Verification items for the finished model (mm, model axes). Face numbers are marked on the shaded views. Coordinates: 2 decimals unless noted, no trailing zeros. Order: outer loops, then holes, each group sorted by start corner. A loop starts at its lowest first (then second) coordinate and runs counter-clockwise, first axis right, second up.
Q1. Draft check along Z on the marked faces 1, 2 and 3. Enter one of: pulls with the +Z half, pulls with the -Z half, needs draft (parallel to the pull), parting line crosses it, or undercut.
Q2. Cross-section at C-C, the plane z = 37. Record the boundary of the cut face in (x, y).
Q3. Cross-section at A-A, the plane x = -65. Record the boundary of the cut face in (y, z).
Q4. Cross-section at D-D, the plane z = 49.5. Record the boundary of the cut face in (x, y), and give its area (3 significant figures).
Q5. Depth check by flat-ended pin: P1, Ø3, axis at x = -34.3, z = -2.66, coming from the -Y side; P2, Ø8, axis at x = 31, z = -0.5, coming from the +Y side; P3, Ø12, axis at x = -205.5, y = 4, coming from the +Z side; P4, Ø11.5, axis at x = 32.47, z = -2.66, coming from the -Y side. Enter the tip coordinate at first touch or a pass-through.
Q6. Thickness scan on line 1 (Y direction, x = 15, z = -5.5); line 2 (X direction, y = 1, z = 0); line 3 (Z direction, x = -62.5, y = 11.75). Record the ranges inside material, lowest first.
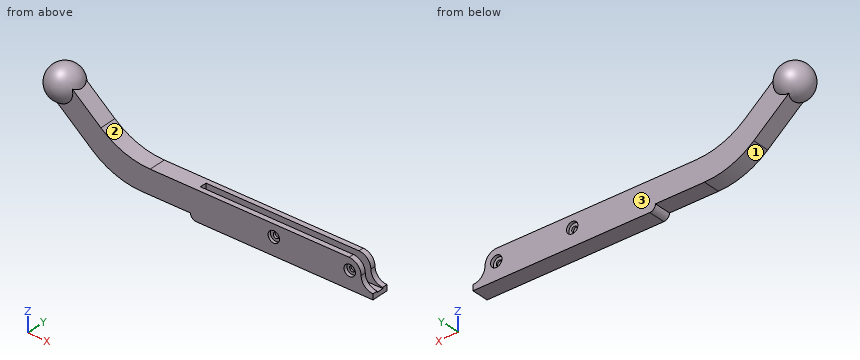
from build123d import *

# Parameters (mm, degrees)
SKETCH_1_W          = 150
SKETCH_1_H          = 21.000000000000004
EXTRUDE_1_DEPTH     = 15
CUT_EXTRUDE_1_DEPTH = 145
SKETCH_3_R          = 5.000000000000004
CUT_EXTRUDE_2_DEPTH = 3
CUT_EXTRUDE_START   = -3
SKETCH_4_R          = 5.000000000000001
CUT_EXTRUDE_3_DEPTH = 3
SKETCH_5_R          = 2.4999999999999987
CUT_EXTRUDE_4_DEPTH = 20
SKETCH_6_R          = 5.000000000000001
CUT_EXTRUDE_5_DEPTH = 20
SKETCH_7_R          = 5.999999999999998
EXTRUDE_2_DEPTH     = 2
SKETCH_8_R          = 6.000000000000003
EXTRUDE_3_DEPTH     = 2
SKETCH_9_R          = 2.500000000000002
CUT_EXTRUDE_6_DEPTH = 20
EXTRUDE_5_DEPTH     = 15
EXTRUDE_6_DEPTH     = 5
FILLET_1_R          = 5
FILLET_2_R          = 10.5
FILLET_3_R          = 67.5
SKETCH_17_W         = 22.000000000000004
SKETCH_17_H         = 5.999999999999995
CUT_EXTRUDE_7_DEPTH = 200


with BuildPart() as part:
    # Sketch 1 → Extrude 1 (new body)
    with BuildSketch(Plane(origin=(0, 0, 0), x_dir=(1, 0, 0), z_dir=(0, 1, 0))):
        with Locations((-32.52921535893155, 2.6552587646076753)):
            Rectangle(SKETCH_1_W, SKETCH_1_H)
    extrude(amount=EXTRUDE_1_DEPTH)

    # Sketch 2 → Cut-Extrude 1 (cut)
    with BuildSketch(Plane(origin=(42.470784641068455, 0, 0), x_dir=(0, 0, -1), z_dir=(1, 0, 0))):
        Polygon((-7.844741235392326, 10.499999999999998), (13.155258764607675, 10.499999999999998), (13.155258764607675, 4.500000000000001), (-7.844741235392326, 4.5), align=None)
    extrude(amount=-CUT_EXTRUDE_1_DEPTH, mode=Mode.SUBTRACT)

    # Sketch 3 → Cut-Extrude 2 (cut)
    with BuildSketch(Plane(origin=(0, 15, 0), x_dir=(1, 0, 0), z_dir=(0, 1, 0))):
        with Locations(Location((32.47078464106845, 2.655258764607675, 0), (0, 0, 270))):
            Circle(SKETCH_3_R)
    extrude(amount=-CUT_EXTRUDE_2_DEPTH, mode=Mode.SUBTRACT)

    # Sketch 4 → Cut-Extrude 3 (cut)
    with BuildSketch(Plane(origin=(0, 0, 0), x_dir=(-1, 0, 0), z_dir=(0, -1, 0)).offset(CUT_EXTRUDE_START)):
        with Locations(Location((-32.47078464106845, 2.655258764607675, 0), (0, 0, 270))):
            Circle(SKETCH_4_R)
    extrude(amount=CUT_EXTRUDE_3_DEPTH, mode=Mode.SUBTRACT)

    # Sketch 5 → Cut-Extrude 4 (cut)
    with BuildSketch(Plane(origin=(0, 3, 0), x_dir=(-1, 0, 0), z_dir=(0, -1, 0))):
        with Locations(Location((-32.47078464106845, 2.655258764607675, 0), (0, 0, 270))):
            Circle(SKETCH_5_R)
    extrude(amount=-CUT_EXTRUDE_4_DEPTH, mode=Mode.SUBTRACT)

    # Sketch 6 → Cut-Extrude 5 (cut)
    with BuildSketch(Plane(origin=(0, 15, 0), x_dir=(1, 0, 0), z_dir=(0, 1, 0))):
        with Locations(Location((-34.295534758931545, 2.655258764607675, 0), (0, 0, 270))):
            Circle(SKETCH_6_R)
    extrude(amount=-CUT_EXTRUDE_5_DEPTH, mode=Mode.SUBTRACT)

    # Sketch 7 → Extrude 2 (add)
    with BuildSketch(Plane(origin=(0, 4.5, 1.9e-16), x_dir=(1, 0, 0), z_dir=(0, 1, 4e-17))):
        with Locations((-34.295534758931545, 2.655258764607675)):
            Circle(SKETCH_7_R)
    extrude(amount=-EXTRUDE_2_DEPTH)

    # Sketch 8 → Extrude 3 (add)
    with BuildSketch(Plane(origin=(0, 10.499999999999998, 0), x_dir=(-1, 0, 0), z_dir=(0, -1, 0))):
        with Locations((34.295534758931545, 2.655258764607675)):
            Circle(SKETCH_8_R)
    extrude(amount=-EXTRUDE_3_DEPTH)

    # Sketch 9 → Cut-Extrude 6 (cut)
    with BuildSketch(Plane(origin=(0, 12.499999999999998, 0), x_dir=(1, 0, 0), z_dir=(0, 1, 0))):
        with Locations(Location((-34.295534758931545, 2.655258764607675, 0), (0, 0, 270))):
            Circle(SKETCH_9_R)
    extrude(amount=-CUT_EXTRUDE_6_DEPTH, mode=Mode.SUBTRACT)



with BuildPart() as body_2:
    # Sketch 12 → Extrude 5 (new body)
    with BuildSketch(Plane(origin=(0, 15, 0), x_dir=(1, 0, 0), z_dir=(0, 1, 0))):
        Polygon((-107.52921535893154, -7.844741235392326), (-167.52921535893154, -7.844741235392335), (-217.32210416166507, -49.62593586501747), (-230.82064396508238, -33.53900255951896), (-175.17259027852143, 13.155258764607666), (-107.52921535893154, 13.155258764607675), align=None)
    extrude(amount=-EXTRUDE_5_DEPTH)

    # Sketch 13 → Revolve 3 (revolve)
    with BuildSketch(Plane(origin=(-151.96584895321814, 0, 127.51448780818791), x_dir=(0.6427876096865401, 0, 0.7660444431189775), z_dir=(-0.7660444431189775, 0, 0.6427876096865401))):
        with BuildLine():
            Line((-112.17628346215061, 22.5), (-112.17628346215061, -7.5))
            ThreePointArc((-112.17628346215061, -7.5), (-97.17628346215061, 7.5), (-112.17628346215061, 22.5))
        make_face()
    revolve(axis=Axis((-224.0713740633737, 22.5, 41.58246921226819), (0, -1, 0)))


with BuildPart() as part_1:
    add(part.part)

    add(body_2.part)  # Extrude 6 merges body 2
    # Sketch 14 → Extrude 6 (add)
    with BuildSketch(Plane(origin=(0, 0, -13.155258764607675), x_dir=(-1, 0, 0), z_dir=(0, 0, -1))):
        Polygon((107.52921535893154, 15), (-52.97078464106847, 14.99999999999998), (-52.97078464106847, -3.99e-14), (107.52921535893154, 0), align=None)
    extrude(amount=EXTRUDE_6_DEPTH)

    # Fillet 1
    fillet_1_edges = [part_1.edges().sort_by_distance(p)[0] for p in [
        (-107.52921535893154, 7.5, -18.155258764607673),
    ]]
    fillet(fillet_1_edges, radius=FILLET_1_R - 0.0001)  # a hair under: the kernel refuses the full size

    # Fillet 2
    fillet_2_edges = [part_1.edges().sort_by_distance(p)[0] for p in [
        (42.470784641068455, 12.75, -13.155258764607675),
    ]]
    fillet(fillet_2_edges, radius=FILLET_2_R - 0.0001)  # a hair under: the kernel refuses the full size
    fillet_2_2_edges = [part_1.edges().sort_by_distance(p)[0] for p in [
        (42.470784641068455, 2.2500000000000004, -13.155258764607675),
    ]]
    fillet(fillet_2_2_edges, radius=FILLET_2_R - 0.0001)  # a hair under: the kernel refuses the full size
    fillet_2_3_edges = [part_1.edges().sort_by_distance(p)[0] for p in [
        (42.470784641068455, 2.25, 7.844741235392326),
    ]]
    fillet(fillet_2_3_edges, radius=FILLET_2_R)
    fillet_2_4_edges = [part_1.edges().sort_by_distance(p)[0] for p in [
        (42.470784641068455, 12.75, 7.844741235392326),
    ]]
    fillet(fillet_2_4_edges, radius=FILLET_2_R)

    # Fillet 3
    fillet_3_edges = [part_1.edges().sort_by_distance(p)[0] for p in [
        (-167.52921535893154, 7.5, 7.844741235392335),
        (-175.17259027852143, 7.5, -13.155258764607666),
    ]]
    fillet(fillet_3_edges, radius=FILLET_3_R)

    # Sketch 17 → Cut-Extrude 7 (cut)
    with BuildSketch(Plane(origin=(-102.52921535893152, 0, 0), x_dir=(0, 0, -1), z_dir=(1, 0, 0))):
        with Locations((3.1552587646076753, 7.500000000000001)):
            Rectangle(SKETCH_17_W, SKETCH_17_H)
    extrude(amount=CUT_EXTRUDE_7_DEPTH, mode=Mode.SUBTRACT)


solid = part_1.part
Check values:
1. face 1: pulls with the -Z half
1. face 2: pulls with the +Z half
1. face 3: needs draft
2. outline: (-211.92, 0) - (-202.28, 0) - (-202.28, 15) - (-211.92, 15) arc R14.28 ccw (long way) to start
3. outline: (0, -18.16) - (15, -18.16) - (15, 7.84) - (10.5, 7.84) - (10.5, -14.16) - (4.5, -14.16) - (4.5, 7.84) - (0, 7.84) - close
4. outline: circle Ø25.48 at (-224.07, 7.5)
4. area: 510 mm2
5. P1: passes through
5. P2: stops at y = 15
5. P3: stops at z = 49.24
5. P4: stops at y = 0
6. line 1: y = 0 to 4.5, 10.5 to 15
6. line 2: x = -190.64 to -38.53, -30.06 to 28.23, 36.71 to 42.13
6. line 3: z = -18.16 to 7.84
